from build123d import *

# Parameters (mm, degrees)
SKETCH1_W               = 70
SKETCH1_H               = 70
BOSS_EXTRUDE1_DEPTH     = 10
SKETCH2_R               = 12
SKETCH2_R_2             = 2
SKETCH2_R_3             = 11.5
CUT_EXTRUDE1_DEPTH      = 10
SKETCH3_W               = 10
SKETCH3_H               = 70
BOSS_EXTRUDE2_DEPTH     = 15
SKETCH4_W               = 10
SKETCH4_H               = 70
BOSS_EXTRUDE3_DEPTH     = 15
SKETCH5_R               = 11.5
SKETCH5_R_2             = 4
BOSS_EXTRUDE4_DEPTH     = 2
SKETCH6_R               = 1.5
SKETCH6_R_2             = 1.648708122
CUT_EXTRUDE3_DEPTH      = 10
BOSS_EXTRUDE5_START     = -10
SKETCH7_R               = 11.986708095
SKETCH7_R_2             = 2
BOSS_EXTRUDE5_DEPTH     = 10
SKETCH8_R               = 12
CUT_EXTRUDE4_DEPTH      = 10
SKETCH9_R               = 2
CUT_EXTRUDE5_DEPTH      = 10
CUT_EXTRUDE7_DEPTH      = 5
SKETCH15_W              = 14
SKETCH15_H              = 70
CUT_EXTRUDE8_DEPTH      = 5
CUT_EXTRUDE9_DEPTH      = 19
CUT_EXTRUDE9_DEPTH_BACK = 48
SKETCH16_R              = 1.5
SKETCH17_R              = 5
CUT_EXTRUDE10_DEPTH     = 19
SKETCH18_W              = 44.558304453
SKETCH18_H              = 39
BOSS_EXTRUDE6_DEPTH     = 5
SKETCH19_R              = 1.5
SKETCH19_R_2            = 5
BOSS_EXTRUDE7_DEPTH     = 3
SKETCH20_W              = 72
SKETCH20_H              = 10
CUT_EXTRUDE11_DEPTH     = 77


with BuildPart() as part:
    # Sketch1 → Boss-Extrude1 (new body)
    with BuildSketch(Plane.XY):
        with Locations((35, 35)):
            Rectangle(SKETCH1_W, SKETCH1_H)
    extrude(amount=BOSS_EXTRUDE1_DEPTH)

    # Sketch2 → Cut-Extrude1 (cut)
    with BuildSketch(Plane.XY.offset(10)):
        with Locations((35, 49)):
            Circle(SKETCH2_R)
        with Locations((19.5, 65)):
            Circle(SKETCH2_R_2)
        with Locations((50.5, 65)):
            Circle(SKETCH2_R_2)
        with Locations((19.5, 34)):
            Circle(SKETCH2_R_2)
        with Locations((50.5, 34)):
            Circle(SKETCH2_R_2)
        with Locations((15, 15)):
            Circle(SKETCH2_R_3)
        with Locations((55, 15)):
            Circle(SKETCH2_R_3)
    extrude(amount=-CUT_EXTRUDE1_DEPTH, mode=Mode.SUBTRACT)

    # Sketch3 → Boss-Extrude2 (add)
    with BuildSketch(Plane.ZY):
        with Locations((5, 35)):
            Rectangle(SKETCH3_W, SKETCH3_H)
    extrude(amount=BOSS_EXTRUDE2_DEPTH)

    # Sketch4 → Boss-Extrude3 (add)
    with BuildSketch(Plane(origin=(70, 0, 0), x_dir=(0, 0, -1), z_dir=(1, 0, 0))):
        with Locations((-5, 35)):
            Rectangle(SKETCH4_W, SKETCH4_H)
    extrude(amount=BOSS_EXTRUDE3_DEPTH)

    # Sketch5 → Boss-Extrude4 (add)
    # profile 1 of 2: a face of its own
    with BuildSketch(Plane.XY.offset(10)):
        with Locations((15, 15)):
            Circle(SKETCH5_R)
        with Locations((15, 15)):
            Circle(SKETCH5_R_2, mode=Mode.SUBTRACT)
    # profile 2 of 2: a face of its own
    with BuildSketch(Plane.XY.offset(10)):
        with Locations((55, 15)):
            Circle(SKETCH5_R)
        with Locations((55, 15)):
            Circle(SKETCH5_R_2, mode=Mode.SUBTRACT)
    extrude(amount=-BOSS_EXTRUDE4_DEPTH)

    # Sketch6 → Cut-Extrude3 (cut)
    with BuildSketch(Plane(origin=(0, 0, 0), x_dir=(-1, 0, 0), z_dir=(0, 0, -1))):
        with Locations((-80, 65)):
            Circle(SKETCH6_R)
        with Locations((-80, 5)):
            Circle(SKETCH6_R)
        with Locations((10, 65)):
            Circle(SKETCH6_R_2)
        with Locations((10, 5)):
            Circle(SKETCH6_R)
    extrude(amount=-CUT_EXTRUDE3_DEPTH, mode=Mode.SUBTRACT)

    # Sketch7 → Boss-Extrude5 (add)
    with BuildSketch(Plane(origin=(0, 0, 0), x_dir=(-1, 0, 0), z_dir=(0, 0, -1)).offset(BOSS_EXTRUDE5_START)):
        with Locations((-35, 49)):
            Circle(SKETCH7_R)
        with Locations((-50.5, 65)):
            Circle(SKETCH7_R_2)
        with Locations((-19.5, 65)):
            Circle(SKETCH7_R_2)
        with Locations((-19.5, 34)):
            Circle(SKETCH7_R_2)
        with Locations((-50.5, 34)):
            Circle(SKETCH7_R_2)
    extrude(amount=BOSS_EXTRUDE5_DEPTH)


with BuildPart() as boss_extrude5_piece_1:
    # of the separate pieces the step leaves, piece 1, a body of its own (boss_extrude5_pieces)
    add(part.part.solids().sort_by_distance((-15, 0, 0))[0])


with BuildPart() as boss_extrude5_piece_2:
    # of the separate pieces the step leaves, piece 2, a body of its own (boss_extrude5_pieces)
    add(part.part.solids().sort_by_distance((23.013291905, 49, 10))[0])


with BuildPart() as cut_extrude4_tool:
    # Sketch8 → Cut-Extrude4 (new body)
    with BuildSketch(Plane(origin=(0, 0, 0), x_dir=(-1, 0, 0), z_dir=(0, 0, -1))):
        with Locations((-33.928692494, 49)):
            Circle(SKETCH8_R)
    extrude(amount=-CUT_EXTRUDE4_DEPTH)


with BuildPart() as boss_extrude5_piece_1_1:
    add(boss_extrude5_piece_1.part)

    # Cut-Extrude4: cut by cut_extrude4_tool
    add(cut_extrude4_tool.part, mode=Mode.SUBTRACT)

    # Sketch9 → Cut-Extrude5 (cut)
    with BuildSketch(Plane(origin=(0, 0, 0), x_dir=(-1, 0, 0), z_dir=(0, 0, -1))):
        with Locations((-49.428692494, 64.5)):
            Circle(SKETCH9_R)
        with Locations((-49.428692494, 33.5)):
            Circle(SKETCH9_R)
        with Locations((-18.428692494, 33.5)):
            Circle(SKETCH9_R)
        with Locations((-18.428692494, 64.5)):
            Circle(SKETCH9_R)
    extrude(amount=-CUT_EXTRUDE5_DEPTH, mode=Mode.SUBTRACT)


with BuildPart() as boss_extrude5_piece_2_1:
    add(boss_extrude5_piece_2.part)

    # Cut-Extrude4: cut by cut_extrude4_tool
    add(cut_extrude4_tool.part, mode=Mode.SUBTRACT)


with BuildPart() as cut_extrude7_tool:
    # Sketch14 → Cut-Extrude7 (new body)
    with BuildSketch(Plane(origin=(0, 0, 0), x_dir=(-1, 0, 0), z_dir=(0, 0, -1))):
        with BuildLine():
            Line((-85, 0), (-85, 70))
            Line((-85, 70), (15, 70))
            Line((15, 70), (15, 0))
            Line((15, 0), (1, 0))
            Line((1, 0), (1, 15))
            ThreePointArc((1, 15), (-15, 31), (-31, 15))
            Line((-31, 15), (-31, 0))
            Line((-31, 0), (-39, 0))
            Line((-39, 0), (-39, 15))
            ThreePointArc((-39, 15), (-55, 31), (-71, 15))
            Line((-71, 15), (-71, 0))
            Line((-71, 0), (-85, 0))
        make_face()
    extrude(amount=-CUT_EXTRUDE7_DEPTH)


with BuildPart() as boss_extrude5_piece_1_2:
    add(boss_extrude5_piece_1_1.part)

    # Cut-Extrude7: cut by cut_extrude7_tool
    add(cut_extrude7_tool.part, mode=Mode.SUBTRACT)

    # Sketch15 → Cut-Extrude8 (cut)
    with BuildSketch(Plane(origin=(0, 0, 5), x_dir=(-1, 0, 0), z_dir=(0, 0, -1))):
        with Locations((-78, 35)):
            Rectangle(SKETCH15_W, SKETCH15_H)
        with Locations((8, 35)):
            Rectangle(SKETCH15_W, SKETCH15_H)
    extrude(amount=-CUT_EXTRUDE8_DEPTH, mode=Mode.SUBTRACT)

    # Sketch16 → Cut-Extrude9 (cut, two sides: drawn at the far end of the back side and taken through both)
    with BuildSketch(Plane(origin=(0, 0, 5), x_dir=(-1, 0, 0), z_dir=(0, 0, -1)).offset(-CUT_EXTRUDE9_DEPTH_BACK)):
        with Locations((-66, 65)):
            Circle(SKETCH16_R)
        with Locations((-66, 5)):
            Circle(SKETCH16_R)
        with Locations((-4, 5)):
            Circle(SKETCH16_R)
        with Locations((-4, 65)):
            Circle(SKETCH16_R)
    extrude(amount=CUT_EXTRUDE9_DEPTH + CUT_EXTRUDE9_DEPTH_BACK, mode=Mode.SUBTRACT)

    # Sketch17 → Cut-Extrude10 (cut)
    with BuildSketch(Plane(origin=(0, 0, 8), x_dir=(-1, 0, 0), z_dir=(0, 0, -1))):
        with Locations((-15, 15)):
            Circle(SKETCH17_R)
        with Locations((-55, 15)):
            Circle(SKETCH17_R)
    extrude(amount=-CUT_EXTRUDE10_DEPTH, mode=Mode.SUBTRACT)



with BuildPart() as boss_extrude5_piece_2_2:
    add(boss_extrude5_piece_2_1.part)

    # Cut-Extrude7: cut by cut_extrude7_tool
    add(cut_extrude7_tool.part, mode=Mode.SUBTRACT)


with BuildPart() as boss_extrude5_piece_1_3:
    add(boss_extrude5_piece_1_2.part)

    add(boss_extrude5_piece_2_2.part)  # Boss-Extrude6 merges Boss-Extrude5 piece 2
    # Sketch18 → Boss-Extrude6 (add)
    with BuildSketch(Plane(origin=(0, 0, 5), x_dir=(-1, 0, 0), z_dir=(0, 0, -1))):
        with Locations((-37.279152227, 50.5)):
            Rectangle(SKETCH18_W, SKETCH18_H)
    extrude(amount=-BOSS_EXTRUDE6_DEPTH)

    # Sketch19 → Boss-Extrude7 (add)
    # profile 1 of 3: a face of its own
    with BuildSketch(Plane.XY.offset(10)):
        with BuildLine():
            Line((71, 0), (71, 15))
            ThreePointArc((71, 15), (66.313708499, 26.313708499), (55, 31))
            Line((55, 31), (15, 31))
            ThreePointArc((15, 31), (3.686291501, 26.313708499), (-1, 15))
            Line((-1, 15), (-1, 0))
            Line((-1, 0), (71, 0))
        make_face()
        with Locations(Location((4, 5, 0), (0, 0, 180))):
            Circle(SKETCH19_R, mode=Mode.SUBTRACT)
        with Locations(Location((15, 15, 0), (0, 0, 180))):
            Circle(SKETCH19_R_2, mode=Mode.SUBTRACT)
        with Locations(Location((66, 5, 0), (0, 0, 180))):
            Circle(SKETCH19_R, mode=Mode.SUBTRACT)
        with Locations(Location((55, 15, 0), (0, 0, 180))):
            Circle(SKETCH19_R_2, mode=Mode.SUBTRACT)
    # profile 2 of 3: a face of its own
    with BuildSketch(Plane.XY.offset(10)):
        with Locations(Location((55, 15, 0), (0, 0, 180))):
            Circle(SKETCH19_R_2)
    # profile 3 of 3: a face of its own
    with BuildSketch(Plane.XY.offset(10)):
        with Locations(Location((15, 15, 0), (0, 0, 180))):
            Circle(SKETCH19_R_2)
    extrude(amount=BOSS_EXTRUDE7_DEPTH)

    # Sketch20 → Cut-Extrude11 (cut)
    with BuildSketch(Plane(origin=(0, 70, 0), x_dir=(1, 0, 0), z_dir=(0, 1, 0))):
        with Locations((35, -5)):
            Rectangle(SKETCH20_W, SKETCH20_H)
    extrude(amount=-CUT_EXTRUDE11_DEPTH, mode=Mode.SUBTRACT)


solid = boss_extrude5_piece_1_3.part
Geometry check sheet. Reference: the model listing, model coordinates, mm. Round coordinates to 2 decimals unless told otherwise and drop trailing zeros. Loops run counter-clockwise (first coordinate to the right, second up) from the corner with the lowest first, then second, coordinate; pieces in that order, holes last.
Item 1: Mould release check, pull along X, two halves, no side actions. Record for faces 1 (the cylindrical face through (64.57, 4.55, 11.48)), 2 (the flat face through (34, 0, 11)), 3 (the cylindrical face through (66.437, 26.189, 11.479)), 4 (the cylindrical face through (2.57, 4.55, 11.48)): pulls with the +X half, pulls with the -X half, needs draft (parallel to the pull), parting line crosses it, or undercut.
Item 2: Thickness scan on line 1 (X direction, y = 5, z = 11.55); line 2 (Y direction, x = 4, z = 11.95); line 3 (Y direction, x = 65.5, z = 11.4). Record the ranges inside material, lowest first.
Item 3: Gauge pin test, flat ends, axial feed: pin 1 (5 mm diameter, centred on x = 66, y = 5, fed in from +Z); pin 2 (1.5 mm diameter, centred on y = 16.5, z = 12.5, fed in from -X). Record the tip position at first contact, or that the pin passes through.
Item 4: Cross-section at C-C on x = 66. Record the boundary of the cut face in (y, z).
Item 5: Cross-section at D-D on y = 20. Record the boundary of the cut face in (x, z).
Item 6: Cross-section at A-A on z = 10.9. Record the boundary of the cut face in (x, y).
Item 7: Cross-section at B-B on y = 5. Record the boundary of the cut face in (x, z).
Answer sheet:
1. face 1: undercut
1. face 2: needs draft
1. face 3: pulls with the +X half
1. face 4: undercut
2. line 1: x = -1 to 2.5, 5.5 to 64.5, 67.5 to 71
2. line 2: y = 0 to 3.5, 6.5 to 26.62
2. line 3: y = 0 to 3.59, 6.41 to 27.07
3. pin 1: stops at z = 13
3. pin 2: stops at x = -0.98
4. outline: (0, 10) - (3.5, 10) - (3.5, 13) - (0, 13) - close; (6.5, 10) - (26.62, 10) - (26.62, 13) - (6.5, 13) - close
5. outline: (-0.2, 10) - (70.2, 10) - (70.2, 13) - (-0.2, 13) - close
6. outline: (-1, 0) - (71, 0) - (71, 15) arc R16 ccw to (55, 31) - (15, 31) arc R16 ccw to (-1, 15) - close; hole circle Ø3 at (4, 5); hole circle Ø3 at (66, 5)
7. outline: (-1, 10) - (2.5, 10) - (2.5, 13) - (-1, 13) - close; (5.5, 10) - (64.5, 10) - (64.5, 13) - (5.5, 13) - close; (67.5, 10) - (71, 10) - (71, 13) - (67.5, 13) - close
